```python
from build123d import *

# Parameters (mm, degrees)
BOSS_EXTRUDE2_DEPTH           = 20
CHAMFER2_SIZE                 = 1.5
CHAMFER2_SIZE2                = 2.598076211
SKETCH4_R                     = 1.5
CUT_EXTRUDE1_DEPTH            = 22.185810788
SKETCH6_W                     = 27
SKETCH6_H                     = 27
BOSS_EXTRUDE4_DEPTH           = 2
CIRPATTERN1_COUNT             = 4
CHAMFER2_OF_CIRPATTERN1_SIZE2 = 1.5
CHAMFER2_OF_CIRPATTERN1_SIZE  = 2.598076211
SKETCH10_R                    = 1.55
CUT_EXTRUDE3_DEPTH            = 32.272991606
FILLET1_R                     = 10
FILLET2_R                     = 2


with BuildPart() as part:
    # Sketch2 → Boss-Extrude2 (new body)
    with BuildSketch(Plane.XY):
        with BuildLine():
            Line((-2.860520074, 4.832233047), (-5.150943513, 7.122656487))
            ThreePointArc((-5.150943513, 7.122656487), (-5.224256058, 7.491223537), (-4.9118, 7.7))
            Line((-4.9118, 7.7), (-2.8048, 7.7))
            ThreePointArc((-2.8048, 7.7), (-2.235720463, 7.935720463), (-2, 8.5048))
            Line((-2, 8.5048), (-2, 8.7126))
            Line((-2, 8.7126), (2, 8.7126))
            Line((2, 8.7126), (2, 8.5048))
            ThreePointArc((2, 8.5048), (2.235720463, 7.935720463), (2.8048, 7.7))
            Line((2.8048, 7.7), (4.9118, 7.7))
            ThreePointArc((4.9118, 7.7), (5.224256058, 7.491223537), (5.150943513, 7.122656487))
            Line((5.150943513, 7.122656487), (2.860520074, 4.832233047))
            ThreePointArc((2.860520074, 4.832233047), (2.049461702, 4.290301169), (1.092753121, 4.1))
            Line((1.092753121, 4.1), (-1.092753121, 4.1))
            ThreePointArc((-1.092753121, 4.1), (-2.049461702, 4.290301169), (-2.860520074, 4.832233047))
        make_face()
    boss_extrude2 = extrude(amount=-BOSS_EXTRUDE2_DEPTH)

    # Chamfer2
    chamfer2_edges = [part.edges().sort_by_distance(p)[0] for p in [
        (0, 8.7126, -20),
    ]]
    chamfer2_side = [part.faces().sort_by_distance(p)[0] for p in [
        (0, 6.450366022, -20),
    ]]
    chamfer(chamfer2_edges, length=CHAMFER2_SIZE, length2=CHAMFER2_SIZE2, reference=chamfer2_side[0])

    # Sketch4 → Cut-Extrude1 (cut, through all)
    with BuildSketch(Plane(origin=(0, 8.7126, 0), x_dir=(1, 0, 0), z_dir=(0, 1, 0))):
        with Locations(Location((0, 15, 0), (0, 0, 270))):
            Circle(SKETCH4_R)
    cut_extrude1 = extrude(amount=-CUT_EXTRUDE1_DEPTH, mode=Mode.SUBTRACT)

    # Sketch6 → Boss-Extrude4 (add)
    with BuildSketch(Plane.XY):
        with Locations((3.5, 3.5)):
            Rectangle(SKETCH6_W, SKETCH6_H)
    extrude(amount=-BOSS_EXTRUDE4_DEPTH)

    # CirPattern1: Boss-Extrude2, Cut-Extrude1 ×4 about axis
    cirpattern1_axis = Axis((0, 0, 0), (0, 0, 1))
    add([boss_extrude2.rotate(cirpattern1_axis, i * 360 / CIRPATTERN1_COUNT) for i in range(1, CIRPATTERN1_COUNT)])
    add([cut_extrude1.rotate(cirpattern1_axis, i * 360 / CIRPATTERN1_COUNT) for i in range(1, CIRPATTERN1_COUNT)], mode=Mode.SUBTRACT)

    # Chamfer2 of CirPattern1
    chamfer2_of_cirpattern1_edges = [part.edges().sort_by_distance(p)[0] for p in [
        (-8.7126, 0, -20),
        (0, -8.7126, -20),
        (8.7126, 0, -20),
    ]]
    chamfer(chamfer2_of_cirpattern1_edges, length=CHAMFER2_OF_CIRPATTERN1_SIZE, length2=CHAMFER2_OF_CIRPATTERN1_SIZE2)

    # Sketch10 → Cut-Extrude3 (cut, through all)
    with BuildSketch(Plane.XY):
        with Locations((0, 12.727922061)):
            Circle(SKETCH10_R)
        with Locations((12.727922061, 0)):
            Circle(SKETCH10_R)
    extrude(amount=-CUT_EXTRUDE3_DEPTH, mode=Mode.SUBTRACT)

    # Fillet1
    fillet1_edges = [part.edges().sort_by_distance(p)[0] for p in [
        (17, 17, -1),
    ]]
    fillet(fillet1_edges, radius=FILLET1_R)

    # Fillet2
    fillet2_edges = [part.edges().sort_by_distance(p)[0] for p in [
        (-10, -10, -1),
        (-10, 17, -1),
        (17, -10, -1),
    ]]
    fillet(fillet2_edges, radius=FILLET2_R)


solid = part.part
```
Geometry check sheet. Reference: the model listing, model coordinates, mm. A direction names the side the tool comes from. Round coordinates to 2 decimals unless told otherwise and drop trailing zeros. Loops run counter-clockwise (first coordinate to the right, second up) from the corner with the lowest first, then second, coordinate; pieces in that order, holes last. Notation, with made-up numbers: (69, 24.5) - (88, 24.5) arc R25 cw to (88, 52.5) - close; hole circle Ø6 at (30, -4.75). An arc over 180 degrees is marked (long way). Write item = value, one per line. Start each with the question number.
1. Mould release check, pull along Y, two halves, no side actions. Record for faces 4 (the face through (4, -7.7, -10)), 5 (the face through (2.062, 4.296, -10.874)), 6 (the face through (7.785, 0.073, -19.008)), 7 (the face through (3, 4, -2)): released by +Y, released by -Y, zero draft, split by the parting line, or undercut.
2. Depth check by flat-ended pin: pin 1 (1.1 mm diameter, centred on y = 3.5, z = -10, fed in from -X); pin 2 (1.7 mm diameter, centred on x = -3.5, z = -8, fed in from -Y) (3 decimals); pin 3 (1.1 mm diameter, centred on x = 0.5, z = -18, fed in from +Y). Enter the tip coordinate at first touch or a pass-through.
3. Thickness scan on line 1 (Y direction, x = 0, z = -1.1); line 2 (Z direction, x = 0, y = -6.2); line 3 (X direction, y = 1, z = -7). Record the ranges inside material, lowest first.
4. Section check C-C on x = 12.75. Enter the section's corners in (y, z), then the cut area to 3 significant figures.
5. Set-up check for faces 1 (the face through (7.93, 2.24, -10.46)), 2 (the face through (-8.713, 0, -10)), 3 (the face through (-7.93, -2.24, -10.46)): record each of +Z, -Z, +X, -X, +Y, -Y from which the full face is reachable in a straight line by a thin tool's end or side.
6. Section check A-A on y = 0. Enter the section's corners in (x, z), then the cut area to 3 significant figures.
7. Section check D-D on z = -15. Give the number of separate pieces and of enclosed holes in the cut face, then the cut area to 3 significant figures.
Working result:
q1.face_4 = released by -Y
q1.face_5 = undercut
q1.face_6 = zero draft
q1.face_7 = undercut
q2.pin_1 = -7.7
q2.pin_2 = -7.715
q2.pin_3 = 8.68
q3.line_1 = -10 to 11.18, 14.28 to 17
q3.line_2 = -20 to -16.5, -13.5 to 0
q3.line_3 = -8.71 to -4.1, 4.1 to 8.71
q4.outline = (-10, -2) - (-1.55, -2) - (-1.55, 0) - (-10, 0) - close; (1.55, -2) - (15.18, -2) - (15.18, 0) - (1.55, 0) - close
q4.area = 44.2 mm^2
q5.face_1 = -Z, +X, +Y
q5.face_2 = -Z, -X, +Y, -Y
q5.face_3 = -Z, -X, -Y
q6.outline = (-10, -2) - (-8.71, -2) - (-8.71, -13.5) - (-4.1, -13.5) - (-4.1, -2) - (4.1, -2) - (4.1, -13.5) - (8.71, -13.5) - (8.71, -2) - (11.18, -2) - (11.18, 0) - (-10, 0) - close; (-8.71, -17.4) - (-7.21, -20) - (-4.1, -20) - (-4.1, -16.5) - (-8.71, -16.5) - close; (4.1, -20) - (7.21, -20) - (8.71, -17.4) - (8.71, -16.5) - (4.1, -16.5) - close; (14.28, -2) - (17, -2) - (17, 0) - (14.28, 0) - close
q6.area = 182 mm^2
q7.separate_pieces = 8
q7.enclosed_holes = 0
q7.area = 72.9 mm^2
